Verification items for the finished model (mm, model axes). A direction names the side the tool comes from. Give positions to 0.01 mm unless a question says otherwise; leave off trailing zeros. Write each loop counter-clockwise with the first axis right and the second up, starting at its lowest first coordinate (ties: lowest second). Pieces come first, ordered by that corner, then holes. Notation, with made-up numbers: (8.5, -2) -> (41.5, -2) arc R16 cw to (41.5, 8) -> close; hole circle Ø8 at (56, -10). An arc over 180 degrees is marked (long way). Write item = value, one per line.
Autodesk Inventor part; units mm, degrees
ref_plane "YZ Plane" through (0, 0, 0) normal (1, 0, 0) x (0, 1, 0)
ref_plane "XZ Plane" through (0, 0, 0) normal (0, 1, 0) x (-1, 0, 0)
ref_plane "XY Plane" through (0, 0, 0) normal (0, 0, 1) x (1, 0, 0)
sketch "Sketch1" plane through (0, 0, 0) normal (0, 0, 1) x (1, 0, 0)
  circle A0 centre (0, 0) radius 8
  dimension "d0" = 16
extrude "Extrusion1" add sketch "Sketch1" along normal blind 20.65
chamfer "Chamfer1" distance 0.5 angle 45 1 edges at (-8, 0, 0)
sketch "Sketch2" plane through (0, 0, 20.65) normal (0, 0, 1) x (1, 0, 0)
  circle A0 centre (0, 0) radius 8
  line L0 (3.4803, 5.9906) -> (6.9282, -0.0187)
  line L1 (6.9282, -0.0187) -> (3.4479, -6.0093)
  line L2 (3.4479, -6.0093) -> (-3.4803, -5.9906)
  line L3 (-3.4803, -5.9906) -> (-6.9282, 0.0187)
  line L4 (-6.9282, 0.0187) -> (-3.4479, 6.0093)
  line L5 (-3.4479, 6.0093) -> (3.4803, 5.9906)
  line L6 (0, 0) -> (3.4803, 5.9906)
  line L7 (0, 0) -> (-3.4479, 6.0093)
  line L8 (-6.9282, 0.0187) -> (0, 0)
  line L9 (-3.4803, -5.9906) -> (0, 0)
  line L10 (3.4479, -6.0093) -> (0, 0)
  line L11 (6.9282, -0.0187) -> (0, 0)
  dimension "d9" = 12
extrude "Extrusion2" add sketch "Sketch2" along normal blind 6.3 contours L6 L7 L5 | L0 L11 L6 | L1 L10 L11 | L7 L8 L4 | L9 L3 L8 | L10 L2 L9
sketch "Sketch3" plane through (0, 0, 0) normal (0, 0, -1) x (-1, 0, 0)
  circle A0 centre (0, 0) radius 2.05
  dimension "d10" = 4.1
extrude "Extrusion3" cut sketch "Sketch3" against normal through all
sketch "Sketch4" plane through (0, 0, 0) normal (0, 0, -1) x (-1, 0, 0)
  circle A0 centre (0, 0) radius 3.1
  dimension "d16" = 6.2
extrude "Extrusion4" cut sketch "Sketch4" against normal blind 20
chamfer "Chamfer3" distance 0.5 angle 45 1 edges at (3.1, 0, 0)
sketch "Sketch5" plane through (0, 0, 0) normal (1, 0, 0) x (0, 1, 0)
  circle A0 centre (0, 6.5) radius 2.4
  line L0 (7.5, 0) -> (-7.5, 0)
  line L1 (-3.6, 0) -> (3.6, 0)
  point P0 (0, 0)
  dimension "d22" = 4.8
  dimension "d23" = 6.5
extrude "Extrusion5" cut sketch "Sketch5" against normal blind 10
properties part number "MotorToHexKey"
Item 1: Mould release check, pull along X, two halves, no side actions. Record for faces 6 (the cylindrical face through (-4.94, 2.29, 7.22)), 7 (the flat face through (-2, -1, 20)), 8 (the flat face through (5.212, -2.972, 23.756)): +X half, -X half, draft (parallel to the pull), parting line (faces both ways), or undercut.
Response values:
face_6 = draft
face_7 = undercut
face_8 = +X half
Item 2: Sectioned sample at A-A on z = 23. Record the cut outline in (x, y).
Response values:
outline = (-6.93, 0.02) -> (-3.48, -5.99) -> (3.45, -6.01) -> (6.93, -0.02) -> (3.48, 5.99) -> (-3.45, 6.01) -> close; hole circle Ø4.1 at (0, 0)
Item 3: Set-up check for faces 1 (the flat face through (-6, -2, 20.65)), 2 (the cylindrical face through (3.1, 0.1, 10.1)), 3 (the flat face through (5.18, 3.03, 23.76)), 4 (the flat face through (-5.18, -3.03, 23.76)), 5 (the flat face through (-5.212, 2.972, 23.756)): record each of +Z, -Z, +X, -X, +Y, -Y from which the full face is reachable in a straight line by a thin tool's end or side.
Response values:
face_1 = +Z
face_2 = -Z
face_3 = +Z, +X, +Y
face_4 = +Z, -X, -Y
face_5 = +Z, -X, +Y
Item 4: Sectioned sample at B-B on x = 0. Record the cut outline in (y, z), then the cut area to 3 significant figures.
Response values:
outline = (-8, 0.5) -> (-7.5, 0) -> (-3.6, 0) -> (-3.1, 0.5) -> (-3.1, 20) -> (-2.05, 20) -> (-2.05, 26.95) -> (-6, 26.95) -> (-6, 20.65) -> (-8, 20.65) -> close; (2.05, 20) -> (3.1, 20) -> (3.1, 0.5) -> (3.6, 0) -> (7.5, 0) -> (8, 0.5) -> (8, 20.65) -> (6, 20.65) -> (6, 26.95) -> (2.05, 26.95) -> close
area = 253 mm^2
Item 5: Material ranges on line 1 (Z direction, x = -6.5, y = 0); line 2 (Y direction, x = 0, z = 10); line 3 (Y direction, x = -5.75, z = 6.5), recorded low to high.
Response values:
line_1 = 0 to 4.1, 8.9 to 26.95
line_2 = -8 to -3.1, 3.1 to 8
line_3 = -5.56 to -2.4, 2.4 to 5.56
Item 6: Sectioned sample at C-C on y = -1.25. Give the number of separate pieces and of enclosed holes in the cut face, then the cut area to 3 significant figures.
Response values:
separate_pieces = 3
enclosed_holes = 0
area = 247 mm^2
Item 7: Sectioned sample at D-D on z = 17. Record the cut outline in (x, y), then the cut area to 3 significant figures.
Response values:
outline = circle Ø16 at (0, 0); hole circle Ø6.2 at (0, 0)
area = 171 mm^2
Item 8: Go/stop test with flat-tipped pins: P1, Ø4, axis at x = 3, z = 22.5, coming from the -Y side; P2, Ø5, axis at x = -1, y = 0, coming from the -Z side; P3, Ø4.5, axis at x = 0, y = 0, coming from the +Z side; P4, Ø4, axis at y = -5.5, z = 5.5, coming from the +X side. Record where each tip stops, or that it passes through.
Response values:
P1 = -7.68
P2 = 0.1
P3 = 26.95
P4 = 7.19
